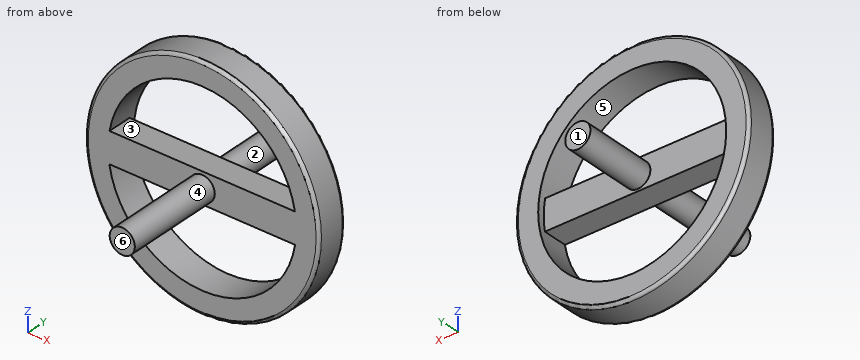
```python
from build123d import *

# Parameters (mm, degrees)
F0_R     = 30.099
F1_DEPTH = 8.128
F2_R     = 24.216053
F3_DEPTH = 25.4
F4_W     = 54.685762
F4_H     = 7.879252
F5_DEPTH = 6.35
F6_R     = 3.239592
F7_DEPTH = 25.4
F8_DEPTH = 25.4
F9_R     = 0.762


with BuildPart() as f1:
    # F0 (on Front) → F1 (new body)
    with BuildSketch(Plane.XZ):
        Circle(F0_R)
    extrude(amount=F1_DEPTH)

    # F2 (on face) → F3 (cut)
    with BuildSketch(Plane.XZ.offset(8.128)):
        Circle(F2_R)
    extrude(amount=-F3_DEPTH, mode=Mode.SUBTRACT)

    # F4 (on face) → F5 (join)
    with BuildSketch(Plane.XZ.offset(8.128)):
        with Locations((-1.039022, 0.136772)):
            Rectangle(F4_W, F4_H)
    extrude(amount=-F5_DEPTH)

    # F6 (on face) → F7 (join)
    with BuildSketch(Plane.XZ.offset(8.128)):
        Circle(F6_R)
    extrude(amount=F7_DEPTH)

    # F6 (on face) → F8 (join)
    with BuildSketch(Plane.XZ.offset(8.128)):
        Circle(F6_R)
    extrude(amount=-F8_DEPTH)

    # F9
    f9_edges = [f1.edges().sort_by_distance(p)[0] for p in [
        (-30.099, 0, 0),
        (-30.099, -8.128, 0),
    ]]
    fillet(f9_edges, radius=F9_R)


solid = f1.part
```
Work out the finished part from the listing and answer in its coordinate system (mm). Face numbers are marked on the shaded views. A direction names the side the tool comes from. Coordinates: 2 decimals unless noted, no trailing zeros. Write each loop counter-clockwise with the first axis right and the second up, starting at its lowest first coordinate (ties: lowest second). Pieces come first, ordered by that corner, then holes. Notation, with made-up numbers: (45.5, -27.5) - (49.5, -27.5) arc R12 ccw to (49.5, -5.5) - close; hole circle Ø11 at (-35, -29). An arc over 180 degrees is marked (long way). Answer as a JSON object with one key per item and string values.
Q1. Find section A-A (x = 0). Write down the section's boundary in (y, z).
Results list:
{"outline": "(-33.53, -3.24) - (-8.13, -3.24) - (-8.13, -3.8) - (-1.78, -3.8) - (-1.78, -3.24) - (17.27, -3.24) - (17.27, 3.24) - (-1.78, 3.24) - (-1.78, 4.08) - (-8.13, 4.08) - (-8.13, 3.24) - (-33.53, 3.24) - close; (-8.13, -29.34) arc R0.76 ccw to (-7.37, -30.1) - (-0.76, -30.1) arc R0.76 ccw to (0, -29.34) - (0, -24.22) - (-8.13, -24.22) - close; (-8.13, 24.22) - (0, 24.22) - (0, 29.34) arc R0.76 ccw to (-0.76, 30.1) - (-7.37, 30.1) arc R0.76 ccw to (-8.13, 29.34) - close"}
Q2. Given pin 1 Ø3 at (y, z) = (-3.5, 4.5) entering from -X; pin 2 Ø7 at (x, y) = (6.5, -5) entering from +Z; pin 3 Ø3 at (x, z) = (-18, -24) entering from +Y, each flat-ended and moving along its own axis, determine where each tip first touches the part or whether it passes through.
Results list:
{"pin 1": "stops at x = -29.95", "pin 2": "stops at z = 29.95", "pin 3": "stops at y = 0"}
Q3. Find section C-C (y = 2.5). Write down the section's boundary in (x, z).
Results list:
{"outline": "circle Ø6.48 at (0, 0)"}
Q4. Consider L1, parallel to Z at x = 0, y = -1.5; L2, parallel to Z at x = 0, y = -5.75; L3, parallel to Y at x = 18, z = -3.5. Determine where each line is inside the solid, lowest interval first. Write a range as from..to.
Results list:
{"L1": "z = -30.1..-24.22, -3.24..3.24, 24.22..30.1", "L2": "z = -30.1..-24.22, -3.8..4.08, 24.22..30.1", "L3": "y = -8.13..-1.78"}
Q5. Find section D-D (x = 21). State how many separate pieces and enclosed holes the cut face has, plus the area to 3 significant figures.
Results list:
{"separate pieces": "3", "enclosed holes": "0", "area": "204 mm^2"}
Q6. Which of the six approach directions +Z, -Z, +X, -X, +Y, -Y give full straight-line access (tool end or side, diameter ignored) to the marked faces 1, 2 and 3?
Results list:
{"face 1": "+Z, -Z, +X, -X, +Y", "face 2": "+Y", "face 3": "+Y, -Y"}
Q7. For a pull along X with two mould halves and no side action, classify the marked faces 4, 5 and 6 as pulls with the +X half, pulls with the -X half, needs draft (parallel to the pull), parting line crosses it, or undercut.
Results list:
{"face 4": "parting line crosses it", "face 5": "undercut", "face 6": "needs draft"}
Q8. Find section B-B (z = 0). Write down the section's boundary in (x, y).
Results list:
{"outline": "(-30.1, -7.37) arc R0.76 ccw to (-29.34, -8.13) - (-3.24, -8.13) - (-3.24, -33.53) - (3.24, -33.53) - (3.24, -8.13) - (29.34, -8.13) arc R0.76 ccw to (30.1, -7.37) - (30.1, -0.76) arc R0.76 ccw to (29.34, 0) - (24.22, 0) - (24.22, -1.78) - (3.24, -1.78) - (3.24, 17.27) - (-3.24, 17.27) - (-3.24, -1.78) - (-24.22, -1.78) - (-24.22, 0) - (-29.34, 0) arc R0.76 ccw to (-30.1, -0.76) - close"}
